```python
from build123d import *

# Parameters (mm, degrees)
SKETCH1_R           = 3.7
BOSS_EXTRUDE1_DEPTH = 3
SKETCH3_R           = 4
BOSS_EXTRUDE3_DEPTH = 20
BOSS_EXTRUDE5_DEPTH = 30
CUT_EXTRUDE1_REACH  = 89.631
SKETCH6_R           = 5
SKETCH6_R_2         = 2
SKETCH8_W           = 3
SKETCH8_H           = 30
BOSS_EXTRUDE6_DEPTH = 12.5


with BuildPart() as part:
    # Sketch1 → Boss-Extrude1 (new body)
    with BuildSketch(Plane(origin=(0, 0, 0), x_dir=(1, 0, 0), z_dir=(0, 1, 0))):
        with BuildLine():
            Line((-37.5, -21), (-37.5, 21))
            ThreePointArc((-37.5, 21), (-33.106601718, 31.606601718), (-22.5, 36))
            Line((-22.5, 36), (22.5, 36))
            ThreePointArc((22.5, 36), (33.106601718, 31.606601718), (37.5, 21))
            Line((37.5, 21), (37.5, -21))
            ThreePointArc((37.5, -21), (33.106601718, -31.606601718), (22.5, -36))
            Line((22.5, -36), (-22.5, -36))
            ThreePointArc((-22.5, -36), (-33.106601718, -31.606601718), (-37.5, -21))
        make_face()
        with Locations(Location((0, 21, 0), (0, 0, 270))):
            Circle(SKETCH1_R, mode=Mode.SUBTRACT)
        with Locations(Location((-20, -21, 0), (0, 0, 270))):
            Circle(SKETCH1_R, mode=Mode.SUBTRACT)
        with Locations(Location((20, -21, 0), (0, 0, 270))):
            Circle(SKETCH1_R, mode=Mode.SUBTRACT)
    extrude(amount=BOSS_EXTRUDE1_DEPTH)

    # Sketch3 → Boss-Extrude3 (add)
    with BuildSketch(Plane(origin=(0, 3, -40.87670084), x_dir=(-1, 0, 0), z_dir=(0, 1, 0))):
        with Locations(Location((-27.5, 27.62670084, 0), (0, 0, 90))):
            Circle(SKETCH3_R)
        with Locations(Location((27.5, 54.12670084, 0), (0, 0, 90))):
            Circle(SKETCH3_R)
        with Locations(Location((-27.5, 54.12670084, 0), (0, 0, 90))):
            Circle(SKETCH3_R)
        with Locations(Location((27.5, 27.62670084, 0), (0, 0, 90))):
            Circle(SKETCH3_R)
    extrude(amount=BOSS_EXTRUDE3_DEPTH)

    # Sketch5 → Boss-Extrude5 (add)
    with BuildSketch(Plane(origin=(0, 3, 0), x_dir=(1, 0, 0), z_dir=(0, 1, 0))):
        Polygon((24, -63.5), (24, -36), (24, -33), (-21, -33), (-21, -36), (21, -36), (21, -63.5), align=None)
    extrude(amount=BOSS_EXTRUDE5_DEPTH)

    # Sketch6 → Cut-Extrude1 (cut, up to next)
    with BuildSketch(Plane.XY.offset(36), mode=Mode.PRIVATE) as cut_extrude1_sk1:
        with Locations((0, 18)):
            Circle(SKETCH6_R)
    cut_extrude1_tool1 = extrude(cut_extrude1_sk1.sketch, amount=-CUT_EXTRUDE1_REACH, mode=Mode.PRIVATE) & part.part
    # Sketch6 → Cut-Extrude1 (cut, up to next)
    with BuildSketch(Plane.XY.offset(36), mode=Mode.PRIVATE) as cut_extrude1_sk2:
        with Locations((-17.5, 26)):
            Circle(SKETCH6_R_2)
    cut_extrude1_tool2 = extrude(cut_extrude1_sk2.sketch, amount=-CUT_EXTRUDE1_REACH, mode=Mode.PRIVATE) & part.part
    # Sketch6 → Cut-Extrude1 (cut, up to next)
    with BuildSketch(Plane.XY.offset(36), mode=Mode.PRIVATE) as cut_extrude1_sk3:
        with Locations((17.5, 26)):
            Circle(SKETCH6_R_2)
    cut_extrude1_tool3 = extrude(cut_extrude1_sk3.sketch, amount=-CUT_EXTRUDE1_REACH, mode=Mode.PRIVATE) & part.part
    add(cut_extrude1_tool1.solids().sort_by_distance((0, 18, 36))[0], mode=Mode.SUBTRACT)
    add(cut_extrude1_tool2.solids().sort_by_distance((-17.5, 26, 36))[0], mode=Mode.SUBTRACT)
    add(cut_extrude1_tool3.solids().sort_by_distance((17.5, 26, 36))[0], mode=Mode.SUBTRACT)

    # Sketch8 → Boss-Extrude6 (add)
    with BuildSketch(Plane.ZY.offset(-21)):
        with Locations((62, 18)):
            Rectangle(SKETCH8_W, SKETCH8_H)
    extrude(amount=BOSS_EXTRUDE6_DEPTH)


solid = part.part
```
Here's how the part is built. I have some questions about the finished solid (model axes, mm). A direction names the side the tool comes from. Coordinates: 2 decimals unless noted, no trailing zeros. Write each loop counter-clockwise with the first axis right and the second up, starting at its lowest first coordinate (ties: lowest second). Pieces come first, ordered by that corner, then holes. Notation, with made-up numbers: (78.25, -24) - (127.25, -24) arc R17 cw to (127.25, 3) - close; hole circle Ø3 at (47, -32.5). An arc over 180 degrees is marked (long way). One line per item, written item: value.
1) I need wall thicknesses on line 1 along X through (y, z) = (1, 21); line 2 along Z through (x, y) = (11, 25.5); line 3 along Y through (x, z) = (-17.5, 35.15). Which ranges of each line are inside material? Lowest first, please.
Model answer:
line 1: x = -37.5 to -23.7, -16.3 to 16.3, 23.7 to 37.5
line 2: z = 33 to 36, 60.5 to 63.5
line 3: y = 0 to 24, 28 to 33
2) Suppose I cut it at C-C on x = -17.5. Write out the boundary of the cut face in (y, z).
Model answer:
outline: (0, -36) - (3, -36) - (3, 18.27) - (0, 18.27) - close; (0, 23.73) - (3, 23.73) - (3, 33) - (24, 33) - (24, 36) - (0, 36) - close; (28, 33) - (33, 33) - (33, 36) - (28, 36) - close
3) Suppose I cut it at D-D on y = 20. Write out the boundary of the cut face in (x, z).
Model answer:
outline: circle Ø8 at (-27.5, -13.25); circle Ø8 at (-27.5, 13.25); (-21, 33) - (-4.58, 33) - (-4.58, 36) - (-21, 36) - close; (4.58, 33) - (24, 33) - (24, 63.5) - (8.5, 63.5) - (8.5, 60.5) - (21, 60.5) - (21, 36) - (4.58, 36) - close; circle Ø8 at (27.5, -13.25); circle Ø8 at (27.5, 13.25)
4) We'd pull the mould along X, two halves only. Please class faces 1 (the cylindrical face through (32.99, 1.48, -31.72)), 2 (the flat face through (1, 0, -1)), 3 (the cylindrical face through (17.066, 24.048, 34.521)): pulls with the +X half, pulls with the -X half, needs draft (parallel to the pull), parting line crosses it, or undercut.
Model answer:
face 1: pulls with the +X half
face 2: needs draft
face 3: undercut
5) I'm going to push flat-ended pins straight in: P1, Ø2.5, axis at x = -26.5, z = -14.5, coming from the +Y side; P2, Ø19.5, axis at y = 21, z = 54, coming from the -X side; P3, Ø3.5, axis at y = 21, z = 34.5, coming from the -X side. Where does each tip first touch, or does it pass through?
Model answer:
P1: stops at y = 23
P2: stops at x = 8.5
P3: stops at x = -21
6) Suppose I cut it at B-B on z = 13.25. Write out the boundary of the cut face in (x, y).
Model answer:
outline: (-37.5, 0) - (37.5, 0) - (37.5, 3) - (31.5, 3) - (31.5, 23) - (23.5, 23) - (23.5, 3) - (-23.5, 3) - (-23.5, 23) - (-31.5, 23) - (-31.5, 3) - (-37.5, 3) - close
7) Suppose I cut it at A-A on y = 11.5. Write out the boundary of the cut face in (x, z).
Model answer:
outline: circle Ø8 at (-27.5, -13.25); circle Ø8 at (-27.5, 13.25); (-21, 33) - (24, 33) - (24, 63.5) - (8.5, 63.5) - (8.5, 60.5) - (21, 60.5) - (21, 36) - (-21, 36) - close; circle Ø8 at (27.5, -13.25); circle Ø8 at (27.5, 13.25)
8) On a 3-axis mill with a long thin cutter (end or side, diameter ignored), from which of +Z, -Z, +X, -X, +Y, -Y can I reach the whole of each face in a straight line? I mean faces 4 (the flat face through (-27, 23, -13)), 5 (the cylindrical face through (30.2, 12.9, -16.2)), 6 (the flat face through (8.5, 18, 62)). Say none if no direction works.
Model answer:
face 4: +Z, -Z, +X, -X, +Y
face 5: +Y
face 6: +Z, -X, +Y, -Y
